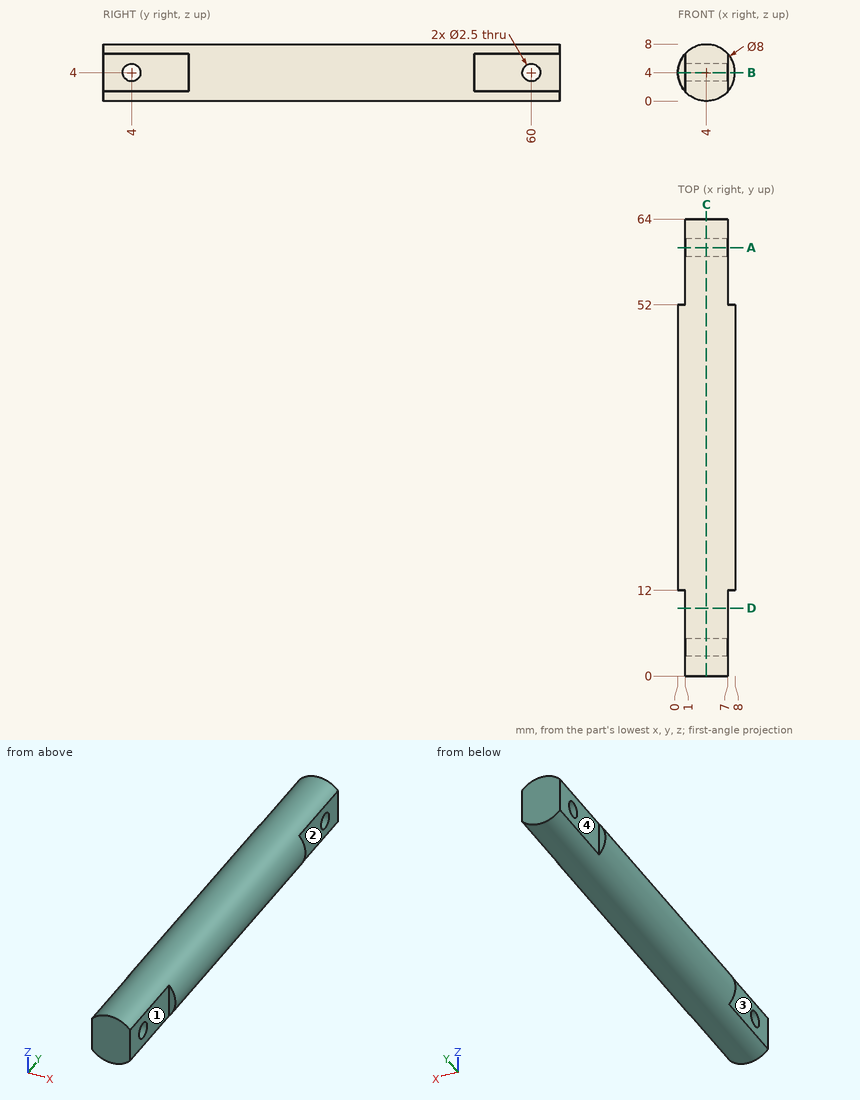
Geometry: see drawing. Coordinates: mm, zero at the bounding-box minimum. A direction names the side the tool comes from. Round coordinates to 2 decimals unless told otherwise and drop trailing zeros. Loops run counter-clockwise (first coordinate to the right, second up) from the corner with the lowest first, then second, coordinate; pieces in that order, holes last. Notation, with made-up numbers: M 83.5,-14.75 L 110.5,-14.75 A22 cw 110.5,17.25 Z; hole C 10.5,59 d5. An arc over 180 degrees is marked long. Use a Markdown table: item, result. Add a question column.
1. Ray query, line 1 along Y through (x, z) = (2.75, 4); line 2 along Y through (x, z) = (6.5, 3.5); line 3 along Z through (x, y) = (1, 27.5). Return the intervals inside material, ascending. Write a range as [from, to].
2. Cut plane A-A, the plane y = 60. Output: boundary loops of the cut face in (x, z), and give its area (3 significant figures).
3. Cut plane C-C, the plane x = 4. Output: boundary loops of the cut face in (y, z).
4. Cut plane D-D, the plane y = 9.5. Output: boundary loops of the cut face in (x, z), and give its area (3 significant figures).
5. Contact query for flat-ended pins moving along their axis: pin 1 (3 mm diameter, centred on x = 7, y = 26, fed in from +Z); pin 2 (3 mm diameter, centred on y = 8.5, z = 2.5, fed in from +X); pin 3 (0.8 mm diameter, centred on x = 0.5, z = 4.5, fed in from -Y). Output: stop coordinate, or through.
6. Set-up query: the marked faces 1, 2, 3 and 4. Return all of +Z, -Z, +X, -X, +Y, -Y with unobstructed straight access to the full face (end or side cutting, diameter ignored); none if empty.
7. Cut plane B-B, the plane z = 4. Output: boundary loops of the cut face in (x, y).
Solution:
| question | item | result |
|---|---|---|
| 1 | line 1 | y = [0, 2.75], [5.25, 58.75], [61.25, 64] |
| 1 | line 2 | y = [0, 2.85], [5.15, 58.85], [61.15, 64] |
| 1 | line 3 | z = [1.35, 6.65] |
| 2 | outline | M 1,1.35 A4 ccw 7,1.35 L 7,2.75 L 1,2.75 Z; M 1,5.25 L 7,5.25 L 7,6.65 A4 ccw 1,6.65 Z |
| 2 | area | 28.0 mm2 |
| 3 | outline | M 0,0 L 64,0 L 64,8 L 0,8 Z; hole C 4,4 d2.5; hole C 60,4 d2.5 |
| 4 | outline | M 1,1.35 A4 ccw 7,1.35 L 7,6.65 A4 ccw 1,6.65 Z |
| 4 | area | 43.0 mm2 |
| 5 | pin 1 | stops at z = 7.71 |
| 5 | pin 2 | stops at x = 7 |
| 5 | pin 3 | stops at y = 12 |
| 6 | face 1 | +Z, -Z, +X, -Y |
| 6 | face 2 | +Z, -Z, +X, +Y |
| 6 | face 3 | +Z, -Z, -X, -Y |
| 6 | face 4 | +Z, -Z, -X, +Y |
| 7 | outline | M 0,12 L 1,12 L 1,5.25 L 7,5.25 L 7,12 L 8,12 L 8,52 L 7,52 L 7,58.75 L 1,58.75 L 1,52 L 0,52 Z; M 1,0 L 7,0 L 7,2.75 L 1,2.75 Z; M 1,61.25 L 7,61.25 L 7,64 L 1,64 Z |
